Can you work these out from the model? Positions are in its coordinate system, mm. A direction names the side the tool comes from. Round coordinates to 2 decimals unless told otherwise and drop trailing zeros. Write each loop counter-clockwise with the first axis right and the second up, starting at its lowest first coordinate (ties: lowest second). Pieces come first, ordered by that corner, then holes. Notation, with made-up numbers: (15.25, 4) - (24.25, 4) arc R13 cw to (24.25, 26) - close; hole circle Ø11 at (30.5, 45.25). An arc over 180 degrees is marked (long way). One line per item, written item: value. Start each with the question number.
(1) I want a section at B-B on y = -4.75. List the corners of the cut face in (x, z) for me, plus the area to 3 significant figures.
(2) If I drill on L1, parallel to Z at x = 0, y = 10.85; L2, parallel to Y at x = -9.25, z = 135, over which ranges is the centre line in solid material (lowest first)? Write a range as from..to.
(3) I want a section at D-D on z = 60. List the corners of the cut face in (x, y) for me, plus the area to 3 significant figures.
(4) On a 3-axis mill with a long thin cutter (end or side, diameter ignored), from which of +Z, -Z, +X, -X, +Y, -Y can I reach the whole of each face in a straight line? I mean faces 1 (the face through (10, 0, 79)), 2 (the face through (0.96, 11.23, 42.31)). Say none if no direction works.
(5) I want a section at C-C on x = 0. Give the number of separate pieces and of enclosed holes in the cut face, plus the area to 3 significant figures.
(6) I want a section at A-A on z = 127.5. List the corners of the cut face in (x, y) for me.
(7) Thinking about a two-plate mould opening in Z: for faces 3 (the face through (-5, -10, 79)), 4 (the face through (0.96, -11.27, 62.31)), 5 (the face through (0, -11, 160)), 6 (the face through (-0.1, 11.2, 77.5)), which applies, +Z half, -Z half, draft (parallel to the pull), parting line (faces both ways), or undercut?
Autodesk Inventor part; units mm, degrees
ref_plane "Work Plane1" through (0, 0, 160) normal (0, 0, -1) x (-1, 0, 0)
ref_plane "Work Plane3" through (-10.5, -12.5, 135.5) normal (0, 0, 1) x (1, 0, 0)
ref_plane "YZ Plane" through (0, 0, 0) normal (1, 0, 0) x (0, 1, 0)
sketch "Sketch1" plane through (0, 0, 0) normal (0, 0, 1) x (1, 0, 0)
  line L0 (-12.5, 12.5) -> (12.5, 12.5)
  line L1 (12.5, 12.5) -> (12.5, -12.5)
  line L2 (12.5, -12.5) -> (-12.5, -12.5)
  line L3 (-12.5, -12.5) -> (-12.5, 12.5)
  line L4 (10, 10) -> (-10, 10)
  line L5 (-10, 10) -> (-10, -10)
  line L6 (-10, -10) -> (10, -10)
  line L7 (10, -10) -> (10, 10)
  point P0 (0, 0)
  dimension "d0" = 25
  dimension "d1" = 25
  dimension "d2" = 12.5
  dimension "d3" = 12.5
  dimension "d4" = 2.5
extrude "Extrusion1" add sketch "Sketch1" along normal blind 1000
fillet "Fillet1" radius 2 4 edges at (12.5, 12.5, 500) (-12.5, 12.5, 500) (-12.5, -12.5, 500) (12.5, -12.5, 500)
ref_plane "Work Plane1" through (0, 0, 160) normal (0, 0, -1) x (-1, 0, 0)
split "Split1" plane through (0, 0, 160) removes the side toward (0, 0, 1)
sketch "Sketch2" plane through (-10.5, 12.5, 0) normal (0, 1, 0) x (1, 0, 0)
  point P0 (10.5, 0)
  point P1 (10.5, -20)
  dimension "d9" = 0
  dimension "d10" = 20
hole "Hole1" at (0, 12.5, 20) direction (0, -1, 0) diameter 5 end through all
pattern_linear "Rectangular Pattern1" count 4 spacing 20 along (0, 0, 1) of "Hole1"
ref_plane "Work Plane3" through (-10.5, -12.5, 135.5) normal (0, 0, 1) x (1, 0, 0)
split "Split3" [suppressed]
equation "\"d0\" = -2 * a + sm_varx_squareBarDimension - tol"
equation "\"d1\" = d0"
equation "\"d4\" = a"
equation "\"d11\" = sm_varx_pinPlate_holeDiameter"
equation "\"d20\" = 0.666667 * sm_varx_squareBarDimension"
equation "\"sm_varx_squareBarThickness\" = 2.5"
equation "\"sm_varx_pinPlate_holeDiameter\" = 5"
equation "\"a\" = sm_varx_squareBarThickness"
equation "\"sm_varx_member_tolerance\" = 0"
equation "\"hoop_angle_z\" = 45deg"
equation "\"hoop_bearing_length\" = 5deg"
equation "\"hoop_bushing12_od\" = -2 * hoop_thickness_large + hoop_width_large + hoop_bushing12_radialInterference"
equation "\"hoop_bushing12_radialInterference\" = 0"
equation "\"hoop_bushing12_thickness\" = -hoop_width_medium + hoop_bushing12_od - 2 * hoop_bushing12_radialInterference"
equation "\"hoop_bushing23_od\" = -2 * hoop_thickness_medium + hoop_width_medium + hoop_bushing23_radialInterference"
equation "\"hoop_bushing23_radialInterference\" = 0"
equation "\"hoop_bushing23_thickness\" = -hoop_width_small + hoop_bushing23_od - 2 * hoop_bushing23_radialInterference"
equation "\"hoop_cable_diam\" = 5"
equation "\"hoop_cable_pulley_diam\" = 22"
equation "\"hoop_tabs_hole\" = 12"
equation "\"hoop_tabs_thickness\" = 6"
equation "\"hoop_thickness_large\" = 4"
equation "\"hoop_thickness_medium\" = 3.2"
equation "\"hoop_thickness_small\" = 2"
equation "\"hoop_width_large\" = 51"
equation "\"hoop_width_medium\" = 33.7"
equation "\"hoop_width_small\" = 25.4"
equation "\"rack_tooth_addendum\" = 5"
equation "\"rack_tooth_dedendum\" = 5"
equation "\"rack_tooth_thickness\" = 5"
equation "\"secure_arm_angle\" = 35deg"
equation "\"secure_arm_radii\" = 9"
equation "\"sm_varx_pinPlate_thickness\" = 5"
equation "\"support_baseClamp_platformLengthBuffer\" = 35"
equation "\"support_baseClamp_platformThickness\" = 15"
equation "\"support_baseClamp_platformWidthBuffer\" = 0"
equation "\"support_baseClamp_sleeveHoleDiameter\" = 12"
equation "\"support_baseClamp_sleeveSweepTerminationAngle\" = 55deg"
equation "\"support_baseClamp_thickness\" = 8"
equation "\"support_frame_endHoleBuffer\" = 45"
equation "\"support_frame_squareBarFillet\" = 2"
equation "\"support_frame_squareBarThickness\" = 5"
equation "\"wheelchair_deployed_height\" = 914"
equation "\"wheelchair_deployed_length\" = 1067"
equation "\"wheelchair_deployed_width\" = 635"
equation "\"wheelchatir_pos_deploy_angle_0\" = 65deg"
equation "\"wheelchatir_pos_store_angle_0\" = 90deg"
equation "\"wheelchatir_pos_deploy_angle_1\" = 20deg"
equation "\"wheelchatir_pos_store_angle_1\" = 20deg"
properties part number "member_vertical_inner" material "Steel, Galvanized"
Established:
1. outline: (-12.5, 0) - (-10, 0) - (-10, 160) - (-12.5, 160) - close; (10, 0) - (12.5, 0) - (12.5, 160) - (10, 160) - close
1. area: 800 mm2
2. L1: 0..17.5, 22.5..37.5, 42.5..57.5, 62.5..77.5, 82.5..160
2. L2: -12.5..-10, 10..12.5
3. outline: (-12.5, -10.5) arc R2 ccw to (-10.5, -12.5) - (-2.5, -12.5) - (-2.5, -10) - (-10, -10) - (-10, 10) - (-2.5, 10) - (-2.5, 12.5) - (-10.5, 12.5) arc R2 ccw to (-12.5, 10.5) - close; (2.5, -12.5) - (10.5, -12.5) arc R2 ccw to (12.5, -10.5) - (12.5, 10.5) arc R2 ccw to (10.5, 12.5) - (2.5, 12.5) - (2.5, 10) - (10, 10) - (10, -10) - (2.5, -10) - close
3. area: 197 mm2
4. face 1: +Z, -Z
4. face 2: +Y, -Y
5. separate pieces: 10
5. enclosed holes: 0
5. area: 700 mm2
6. outline: (-12.5, -10.5) arc R2 ccw to (-10.5, -12.5) - (10.5, -12.5) arc R2 ccw to (12.5, -10.5) - (12.5, 10.5) arc R2 ccw to (10.5, 12.5) - (-10.5, 12.5) arc R2 ccw to (-12.5, 10.5) - close; hole (-10, -10) - (10, -10) - (10, 10) - (-10, 10) - close
7. face 3: draft
7. face 4: undercut
7. face 5: +Z half
7. face 6: undercut
